Input: part model. Units: mm. Frame: model coordinates. A direction names the side the tool comes from. Coordinates: 2 decimals unless noted, no trailing zeros. Write each loop counter-clockwise with the first axis right and the second up, starting at its lowest first coordinate (ties: lowest second). Pieces come first, ordered by that corner, then holes. Notation, with made-up numbers: (33.5, -8) - (89.5, -8) arc R7 ccw to (89.5, -4) - close; hole circle Ø4 at (-4, 27). An arc over 180 degrees is marked (long way). One line per question, with ' | ' between items. Start each with the question number.
1) Section query B-B on z = 2.75. Return loops of the section in (x, y), and give its area (3 significant figures).
2) Draft query along Y for faces 4 (the cylindrical face through (-0.74, -0.59, 4.46)), 5 (the flat face through (-17.5, 0, 0)), 6 (the flat face through (-1.479, -0.74, 1.305)). Return one class per face: released by +Y, released by -Y, zero draft, split by the parting line, or undercut.
3) Reachability of faces 1 (the cylindrical face through (-9.14, 0.54, -2.44)), 2 (the flat face through (0, 0, -2)), 3 (the flat face through (-1.479, -0.76, -1.293)) from +Z, -Z, +X, -X, +Y, -Y: full face, straight path, thin tool, end or side. Return the list, or none.
4) Section query C-C on z = -3.5. Return loops of the section in (x, y), and give its area (3 significant figures).
5) Line query: line 1 (Z direction, x = -7.5, y = 2); line 2 (Y direction, x = -9.5, z = -1.5); line 3 (X direction, y = 3.25, z = -2.75). Output: solid intervals per line, ascending.
6) Section query A-A on z = 0. Return loops of the section in (x, y).
7) First-contact query: P1, Ø3, axis at x = -9, y = -2.5, coming from the +Z side; P2, Ø1, axis at x = -11.5, y = 0, coming from the +Z side; P3, Ø0.9, axis at x = -2, z = 0.5, coming from the -Y side; P4, Ø3.5, axis at y = 0, z = 1, coming from the +X side. Flat tips, straight axial feed; report the tip coordinate or a pass-through.
```python
from build123d import *

# Parameters (mm, degrees)
F0_R     = 4.5
F1_DEPTH = 1.5
F2_R     = 2.5
F3_DEPTH = 16
F4_SIZE  = 0.5
F6_DEPTH = 3


with BuildPart() as f1:
    # F0 (on Right) → F1 (new body)
    with BuildSketch(Plane.YZ):
        Circle(F0_R)
    extrude(amount=-F1_DEPTH)

    # F2 (on face) → F3 (join)
    with BuildSketch(Plane(origin=(-1.5, 0, 0), x_dir=(0, -1, 0), z_dir=(-1, 0, 0))):
        Circle(F2_R)
    extrude(amount=F3_DEPTH)

    # F4
    f4_edges = [f1.edges().sort_by_distance(p)[0] for p in [
        (-17.5, 2.5, 0),
    ]]
    chamfer(f4_edges, length=F4_SIZE)

    # F5 (on face) → F6 (cut)
    with BuildSketch(Plane.YZ):
        Polygon((0, -1.732051), (1.5, -0.866025), (1.5, 0.866025), (0, 1.732051), (-1.5, 0.866025), (-1.5, -0.866025), align=None)
    extrude(amount=-F6_DEPTH, mode=Mode.SUBTRACT)


solid = f1.part
```
Answer key:
1) outline: (-1.5, -3.56) - (0, -3.56) - (0, 3.56) - (-1.5, 3.56) - close | area: 10.7 mm²
2) face 4: split by the parting line | face 5: zero draft | face 6: undercut
3) face 1: -X | face 2: +Z, -Z, +X, +Y, -Y | face 3: +X
4) outline: (-1.5, -2.83) - (0, -2.83) - (0, 2.83) - (-1.5, 2.83) - close | area: 8.49 mm²
5) line 1: -1.5 to 1.5 | line 2: -2 to 2 | line 3: -1.5 to 0
6) outline: (-17.5, -2) - (-17, -2.5) - (-1.5, -2.5) - (-1.5, -4.5) - (0, -4.5) - (0, -1.5) - (-3, -1.5) - (-3, 1.5) - (0, 1.5) - (0, 4.5) - (-1.5, 4.5) - (-1.5, 2.5) - (-17, 2.5) - (-17.5, 2) - close
7) P1: z = 2.29 | P2: z = 2.5 | P3: y = -2.5 | P4: x = 0
